```python
from build123d import *

# Parameters (mm, degrees)
F2_W     = 19.05
F2_H     = 6.35
F3_DEPTH = 12.7
F4_R     = 3.175
F5_DEPTH = 12.7
F7_R     = 3.175
F8_DEPTH = 25.4


with BuildPart() as f1:
    # F0 (on Front) → F1 (revolve)
    with BuildSketch(Plane.XZ):
        with BuildLine():
            add(Edge.make_bspline(
                [(0, -12.065), (9.525, -12.065), (9.525, 0)],
                knots=[3.1415926536, 3.1415926536, 3.1415926536, 4.7123889804, 4.7123889804, 4.7123889804], degree=2, weights=[1, 0.7071067812, 1]))
            ThreePointArc((9.525, 0), (6.7351920908, 6.7351920908), (0, 9.525))
            Line((0, 9.525), (0, -12.065))
        make_face()
    revolve(axis=Axis((0, 0, 2.0303288475), (0, 0, -1)))

    # F2 (on Top) → F3 (cut, symmetric)
    with BuildSketch(Plane.XY):
        with Locations((0, 7.9375)):
            Rectangle(F2_W, F2_H)
        with Locations((0, -7.9375)):
            Rectangle(F2_W, F2_H)
    extrude(amount=F3_DEPTH, both=True, mode=Mode.SUBTRACT)

    # F4 (on Front) → F5 (cut, symmetric)
    with BuildSketch(Plane.XZ):
        Circle(F4_R)
    extrude(amount=F5_DEPTH, both=True, mode=Mode.SUBTRACT)

    # F7 (on offset) → F8 (join)
    with BuildSketch(Plane.XY.offset(-11.43)):
        Circle(F7_R)
    extrude(amount=-F8_DEPTH)


solid = f1.part
```
Check sheet for the modelled part. Datum: model origin and axes. Units: mm. A direction names the side the tool comes from. Give positions to 0.01 mm unless a question says otherwise; leave off trailing zeros. Order: outer loops, then holes, each group sorted by start corner. A loop starts at its lowest first (then second) coordinate and runs counter-clockwise, first axis right, second up. Notation, with made-up numbers: M 7.5,0.5 L 55.5,0.5 A21 cw 55.5,13.5 Z; hole C 86,9.25 d5. An arc over 180 degrees is marked long. Answer in a Markdown table with one row per item.
1) Access from +Z, -Z, +X, -X, +Y, -Y to the whole of each face (thin tool, end or side, straight path). Record for faces 1 (the flat face through (2, 4.762, -3)), 2 (the cylindrical face through (-0.69, -3.1, -23.95)).
Filled sheet:
| item | result |
|---|---|
| face 1 | +Z, -Z, +X, -X, +Y |
| face 2 | -Z |
2) Release check for a two-part mould opening along Z. For faces 3 (the flat face through (0, 0, -36.83)), 4 (the cylindrical face through (-0.69, -0.07, -3.1)), 5 (the flat face through (2, -4.762, -3)) record: +Z half, -Z half, draft (parallel to the pull), parting line (faces both ways), or undercut.
Filled sheet:
| item | result |
|---|---|
| face 3 | -Z half |
| face 4 | undercut |
| face 5 | draft |
3) Thickness scan on L1, parallel to Z at x = 0, y = -0.25 (3 decimals); L2, parallel to Z at x = 1.5, y = -1.75; L3, parallel to X at y = 3.25, z = 2. Record the ranges inside material, lowest first. Write a range as [from, to].
Filled sheet:
| item | result |
|---|---|
| L1 | z = [-36.83, -3.175], [3.175, 9.522] |
| L2 | z = [-36.83, -2.8], [2.8, 9.24] |
| L3 | x = [-8.73, -2.47], [2.47, 8.73] |
4) Cross-section at A-A, the plane z = -27. Enter the section's corners in (x, y) (3 decimals).
Filled sheet:
| item | result |
|---|---|
| outline | C 0,0 d6.35 |
5) Gauge pin test, flat ends, axial feed: P1, Ø2, axis at x = 5, y = 3.5, coming from the +Z side; P2, Ø1.9, axis at x = -0.5, y = -1, coming from the +Z side; P3, Ø3, axis at x = 2, z = -16.5, coming from the +Y side. Record the tip position at first contact, or that the pin passes through.
Filled sheet:
| item | result |
|---|---|
| P1 | stops at z = 8.04 |
| P2 | stops at z = 9.52 |
| P3 | stops at y = 3.14 |
